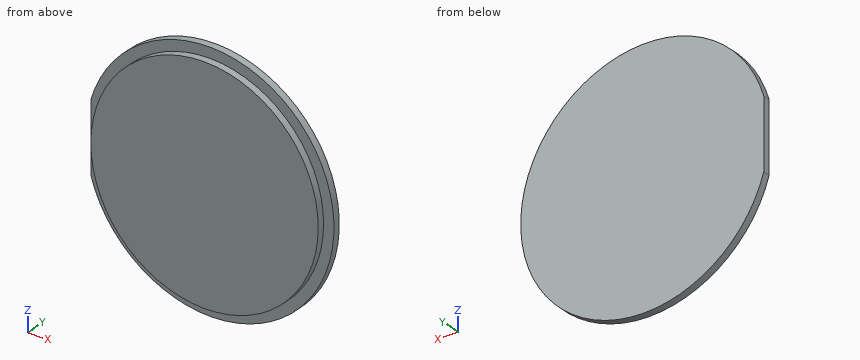
```python
from build123d import *

# Parameters (mm, degrees)
SKETCH_1_R          = 15.9
EXTRUDE_1_DEPTH     = 1
SKETCH_2_R          = 17.35
EXTRUDE_2_DEPTH     = 1
CUT_EXTRUDE_1_DEPTH = 1


with BuildPart() as part:
    # 草图1 → 凸台-拉伸1 (new body)
    with BuildSketch(Plane(origin=(0, 0, 0), x_dir=(1, 0, 0), z_dir=(0, 1, 0))):
        Circle(SKETCH_1_R)
    extrude(amount=EXTRUDE_1_DEPTH)

    # 草图2 → 凸台-拉伸2 (add)
    with BuildSketch(Plane(origin=(0, 1, 0), x_dir=(1, 0, 0), z_dir=(0, 1, 0))):
        Circle(SKETCH_2_R)
    extrude(amount=EXTRUDE_2_DEPTH)

    # 草图3 → 切除-拉伸1 (cut)
    with BuildSketch(Plane.XZ.offset(-1)):
        with BuildLine():
            Line((-16.65, 4.878524367), (-16.65, -4.878524367))
            ThreePointArc((-16.65, -4.878524367), (-17.35, 0), (-16.65, 4.878524367))
        make_face()
    extrude(amount=-CUT_EXTRUDE_1_DEPTH, mode=Mode.SUBTRACT)


solid = part.part
```
Design review of the part built by this model. Coordinates are the model's own, in mm. Give positions to 0.01 mm unless a question says otherwise; leave off trailing zeros. Loops run counter-clockwise (first coordinate to the right, second up) from the corner with the lowest first, then second, coordinate; pieces in that order, holes last. Notation, with made-up numbers: M -27.5,84.5 L 10.5,84.5 A23 cw 10.5,116.5 Z; hole C 7,80.25 d3. An arc over 180 degrees is marked long. Return JSON: item names as keys, results as strings. Group by question number.
Item 1: For probe 1 along X at (y, z) = (0.75, 0.5); probe 2 along X at (y, z) = (0.9, -13.5); probe 3 along Z at (x, y) = (10, 1.6), list the stretches that pass through material, from the lowest coordinate up.
Item 2: We need section B-B (x = 0). Give the boundary of the cut face in (y, z), and give its area (3 significant figures).
Item 3: Insertion check: pin 1 Ø1 at (x, y) = (3.5, 1) entering from -Z; pin 2 Ø10 at (x, z) = (-4, -1) entering from -Y. Each pin has a flat end and moves straight along its axis. Give the tip position at first contact, or say it passes through.
Item 4: We need section A-A (z = 0). Give the boundary of the cut face in (x, y), and give its area (3 significant figures).
Output:
{
 "1": {"probe 1": "x = -15.89 to 15.89", "probe 2": "x = -8.4 to 8.4", "probe 3": "z = -14.18 to 14.18"},
 "2": {"outline": "M 0,-15.9 L 1,-15.9 L 1,-17.35 L 2,-17.35 L 2,17.35 L 1,17.35 L 1,15.9 L 0,15.9 Z", "area": "66.5 mm^2"},
 "3": {"pin 1": "stops at z = -17.09", "pin 2": "stops at y = 0"},
 "4": {"outline": "M -16.65,1 L -15.9,1 L -15.9,0 L 15.9,0 L 15.9,1 L 17.35,1 L 17.35,2 L -16.65,2 Z", "area": "65.8 mm^2"}
}
